Part print with two shaded views. Sizes in mm from the minimum x, y, z corner. A direction names the side the tool comes from. Round coordinates to 2 decimals unless told otherwise and drop trailing zeros. Loops run counter-clockwise (first coordinate to the right, second up) from the corner with the lowest first, then second, coordinate; pieces in that order, holes last. Notation, with made-up numbers: M 83.5,55 L 121.5,55 A25 cw 121.5,74 Z; hole C 15.25,19 d2. An arc over 180 degrees is marked long. Answer as CSV lines item,"result". Start each with the question number.
Item 1: Band-saw the part on C-C (z = 6). Give the cut face in (x, y).
Item 2: Band-saw the part on B-B (x = 3). Give the cut face in (y, z).
Item 3: Which spindle directions (+Z, -Z, +X, -X, +Y, -Y) get a long thin tool onto all of the face, cutting with end or side? Do the marked faces 1, 2 and 3. Say none if no direction does.
Item 4: Band-saw the part on A-A (x = 32). Give the cut face in (y, z).
Item 5: Drop flat-ended pins along their axis: pin 1 Ø8 at (x, y) = (30, 48.5) entering from +Z; pin 2 Ø6 at (y, z) = (26, 38) entering from +X; pin 3 Ø2 at (x, y) = (43, 7.5) entering from +Z; pin 4 Ø12.5 at (x, z) = (41.5, 20) entering from -Y. Give the stop position or say it passes through.
Item 6: Wall check: line 1 (Y direction, x = 32, z = 3); line 2 (Z direction, x = 20.5, y = 25.5); line 3 (Y direction, x = 18.5, z = 25.5). Give the ranges that are in metal, low to high.
Item 7: Band-saw the part on D-D (y = 25). Give the cut face in (x, z), and give its area (3 significant figures).
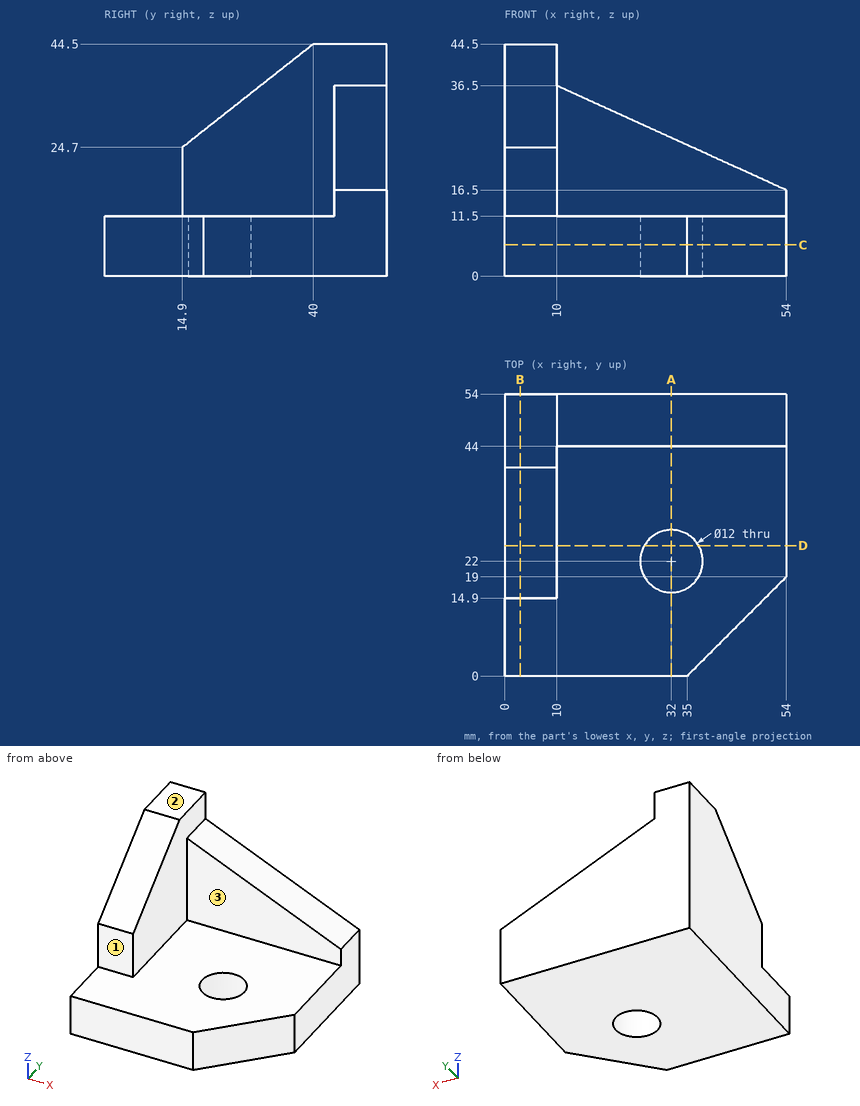
Answer block:
1,outline,"M 0,0 L 35,0 L 54,19 L 54,54 L 0,54 Z; hole C 32,22 d12"
2,outline,"M 0,0 L 54,0 L 54,44.5 L 40,44.5 L 14.9,24.7 L 14.9,11.5 L 0,11.5 Z"
3,face 1,"+Z, +X, -X, -Y"
3,face 2,"+Z, +X, -X, +Y, -Y"
3,face 3,"+Z, +X, -Y"
4,outline,"M 0,0 L 16,0 L 16,11.5 L 0,11.5 Z; M 28,0 L 54,0 L 54,26.5 L 44,26.5 L 44,11.5 L 28,11.5 Z"
5,pin 1,"stops at z = 29.23"
5,pin 2,"passes through"
5,pin 3,"stops at z = 11.5"
5,pin 4,"stops at y = 44"
6,line 1,"y = 0 to 16, 28 to 54"
6,line 2,"z = 0 to 11.5"
6,line 3,"y = 44 to 54"
7,outline,"M 0,0 L 26.8,0 L 26.8,11.5 L 10,11.5 L 10,32.67 L 0,32.67 Z; M 37.2,0 L 54,0 L 54,11.5 L 37.2,11.5 Z"
7,area,"713 mm^2"
